Here's how the part is built. I have some questions about the finished solid (model axes, mm). Face numbers are marked on the shaded views. Coordinates: 2 decimals unless noted, no trailing zeros. Order: outer loops, then holes, each group sorted by start corner. A loop starts at its lowest first (then second) coordinate and runs counter-clockwise, first axis right, second up.
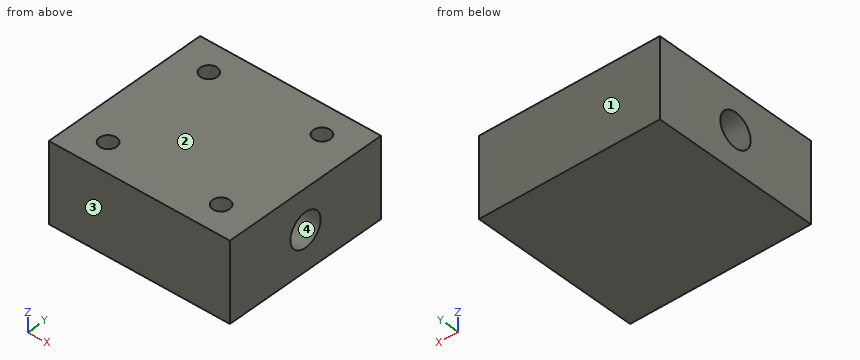
```python
from build123d import *

# Parameters (mm, degrees)
SKETCH_1_W          = 32
SKETCH_1_H          = 30
EXTRUDE_1_DEPTH     = 14
SKETCH_2_R          = 3
CUT_EXTRUDE_1_DEPTH = 33
SKETCH_3_R          = 1.5
CUT_EXTRUDE_2_DEPTH = 3


with BuildPart() as part:
    # 草图1 → 凸台-拉伸1 (new body)
    with BuildSketch(Plane.XY):
        Rectangle(SKETCH_1_W, SKETCH_1_H)
    extrude(amount=EXTRUDE_1_DEPTH)

    # 草图2 → 切除-拉伸1 (cut)
    with BuildSketch(Plane(origin=(16, 0, 0), x_dir=(0, 0, -1), z_dir=(1, 0, 0))):
        with Locations((-7, 0)):
            Circle(SKETCH_2_R)
    extrude(amount=-CUT_EXTRUDE_1_DEPTH, mode=Mode.SUBTRACT)

    # 草图3 → 切除-拉伸2 (cut)
    with BuildSketch(Plane.XY.offset(14)):
        with Locations((-10, 10)):
            Circle(SKETCH_3_R)
        with Locations((10, 10)):
            Circle(SKETCH_3_R)
        with Locations((10, -10)):
            Circle(SKETCH_3_R)
        with Locations((-10, -10)):
            Circle(SKETCH_3_R)
    extrude(amount=-CUT_EXTRUDE_2_DEPTH, mode=Mode.SUBTRACT)


solid = part.part
```
Q1. I need wall thicknesses on L1, parallel to Y at x = -10, z = 11.95; L2, parallel to Y at x = 9.5, z = 7; L3, parallel to Z at x = -11, y = -1.5. Which ranges of each line are inside material? Lowest first, please.
Q2. Will this pin go through, and if not, where does the flat tip stop? pin 1 (1.8 mm diameter, centred on x = -10, y = -10, fed in from +Z).
Q3. If we section it at D-D on z = 11.5: Write out the boundary of the cut face in (x, y), then the cut area to 3 significant figures.
Q4. If we section it at A-A on y = 0: Write out the boundary of the cut face in (x, z).
Q5. We'd pull the mould along Y, two halves only. Please class the marked faces 1, 2, 3 and 4: pulls with the +Y half, pulls with the -Y half, needs draft (parallel to the pull), parting line crosses it, or undercut.
Q6. If we section it at B-B on z = 7: Write out the boundary of the cut face in (x, y), then the cut area to 3 significant figures.
Q7. If we section it at C-C on x = 10: Write out the boundary of the cut face in (y, z).
Reply:
1. L1: y = -15 to -11.5, -8.5 to 8.5, 11.5 to 15
1. L2: y = -15 to -3, 3 to 15
1. L3: z = 0 to 4.4, 9.6 to 14
2. pin 1: stops at z = 11
3. outline: (-16, -15) - (16, -15) - (16, 15) - (-16, 15) - close; hole circle Ø3 at (-10, -10); hole circle Ø3 at (-10, 10); hole circle Ø3 at (10, -10); hole circle Ø3 at (10, 10)
3. area: 932 mm2
4. outline: (-16, 0) - (16, 0) - (16, 4) - (-16, 4) - close; (-16, 10) - (16, 10) - (16, 14) - (-16, 14) - close
5. face 1: pulls with the +Y half
5. face 2: needs draft
5. face 3: pulls with the -Y half
5. face 4: undercut
6. outline: (-16, -15) - (16, -15) - (16, -3) - (-16, -3) - close; (-16, 3) - (16, 3) - (16, 15) - (-16, 15) - close
6. area: 768 mm2
7. outline: (-15, 0) - (15, 0) - (15, 14) - (11.5, 14) - (11.5, 11) - (8.5, 11) - (8.5, 14) - (-8.5, 14) - (-8.5, 11) - (-11.5, 11) - (-11.5, 14) - (-15, 14) - close; hole circle Ø6 at (0, 7)
